```python
from build123d import *

# Parameters (mm, degrees)
SKETCH_R           = 7.5
SKETCH_R_2         = 3.8
PAD_DEPTH          = 30
SKETCH001_W        = 1
SKETCH001_H        = 2
POCKET_DEPTH       = 30
POLARPATTERN_COUNT = 16


with BuildPart() as part:
    # Sketch → Pad (new body)
    with BuildSketch(Plane.XY):
        Circle(SKETCH_R)
        Circle(SKETCH_R_2, mode=Mode.SUBTRACT)
    extrude(amount=PAD_DEPTH)

    # Sketch001 (on Face4 of Pad) → Pocket (cut)
    with BuildSketch(Plane.XY.offset(30)):
        with Locations((0, 4.766962)):
            Rectangle(SKETCH001_W, SKETCH001_H)
    pocket = extrude(amount=-POCKET_DEPTH, mode=Mode.SUBTRACT)

    # PolarPattern: Pocket ×16 about axis
    polarpattern_axis = Axis((0, 0, 30), (0, 0, 1))
    for i in range(1, POLARPATTERN_COUNT):
        add(pocket.rotate(polarpattern_axis, i * 360 / POLARPATTERN_COUNT), mode=Mode.SUBTRACT)


solid = part.part
```
Geometry check sheet. Reference: the model listing, model coordinates, mm. Coordinates: 2 decimals unless noted, no trailing zeros. Loops run counter-clockwise (first coordinate to the right, second up) from the corner with the lowest first, then second, coordinate; pieces in that order, holes last. Notation, with made-up numbers: (14.5, 15.25) - (20.5, 15.25) arc R9 cw to (20.5, 19.25) - close; hole circle Ø7 at (-11.5, 69). An arc over 180 degrees is marked (long way). One line per item, written item: value. Start each with the question number.
(1) Depth check by flat-ended pin: P1, Ø1.5, axis at x = -4, z = 11.5, coming from the -Y side; P2, Ø0.6, axis at y = -4.5, z = 21, coming from the -X side; P3, Ø0.6, axis at x = -5, z = 8, coming from the -Y side. Enter the tip coordinate at first touch or a pass-through.
(2) Cross-section at A-A on y = 0. Enter the section's corners in (x, z), plus the area to 3 significant figures.
(3) Material ranges on line 1 (X direction, y = -5, z = 9.5); line 2 (X direction, y = -4.25, z = 4.5); line 3 (X direction, y = -2.5, z = 6), recorded low to high. Write a range as [from, to].
(4) Mould release check, pull along Y, two halves, no side actions. Record for faces 1 (the flat face through (3, -5, 0)), 2 (the cylindrical face through (-7.493, 0.33, 14.79)), 3 (the flat face through (2.213, -5.325, 15.21)): released by +Y, released by -Y, zero draft, split by the parting line, or undercut.
(5) Cross-section at C-C on y = 6.5. Enter the section's corners in (x, z).
Results below:
1. P1: stops at y = -6.76
1. P2: stops at x = -6.21
1. P3: stops at y = -5.84
2. outline: (-7.5, 0) - (-5.77, 0) - (-5.77, 30) - (-7.5, 30) - close; (5.77, 0) - (7.5, 0) - (7.5, 30) - (5.77, 30) - close
2. area: 104 mm2
3. line 1: x = [-5.59, -2.61], [-1.53, -0.5], [0.5, 1.53], [2.61, 5.59]
3. line 2: x = [-6.18, -3.91], [-3.54, -2.3], [-1.22, -0.5], [0.5, 1.22], [2.3, 3.54], [3.91, 6.18]
3. line 3: x = [-7.07, -5.21], [-4.73, -3.21], [3.21, 4.73], [5.21, 7.07]
4. face 1: zero draft
4. face 2: split by the parting line
4. face 3: undercut
5. outline: (-3.74, 0) - (3.74, 0) - (3.74, 30) - (-3.74, 30) - close
